```python
from build123d import *

# Parameters (mm, degrees)
F0_W     = 10
F0_H     = 20
F1_ANGLE = 180
F2_R     = 0.6542669189
F2_R_2   = 0.5762174249
F2_R_3   = 1.2390393019
F2_R_4   = 1.4098966941
F2_R_5   = 0.189897881
F2_R_6   = 0.6151811848
F2_R_7   = 0.7778029264
F2_R_8   = 0.6623255224
F2_R_9   = 0.6070903234
F2_R_10  = 0.7783808961
F2_R_11  = 0.265053414
F2_R_12  = 0.5177294077
F2_R_13  = 0.5684145952
F2_R_14  = 0.5786464401
F4_DEPTH = 1


# Not quite as in the source:
# - the program builds the solid bodies; features that only make, move or delete a surface that nothing else refers to are left out


with BuildPart() as f1:
    # F0 (on Front) → F1 (revolve)
    with BuildSketch(Plane.XZ):
        with Locations((5, 10)):
            Rectangle(F0_W, F0_H)
        with BuildLine():
            Line((10, 0), (0, 0))
            ThreePointArc((0, 0), (2.9289321881, -7.0710678119), (10, -10))
            Line((10, -10), (10, 0))
        make_face()
        with BuildLine():
            ThreePointArc((10, 30), (2.9289321881, 27.0710678119), (0, 20))
            Line((0, 20), (10, 20))
            Line((10, 20), (10, 30))
        make_face()
    revolve(axis=Axis((10, 0, 10), (0, 0, -1)), revolution_arc=F1_ANGLE)

    # F2 (on face) → F4 (join)
    with BuildSketch(Plane.XZ):
        with Locations((5.6774760596, 22.7308552712)):
            Circle(F2_R)
        with Locations((16.3127072155, 20.606238395)):
            Circle(F2_R_2)
        with Locations((3.6300569773, 15.6070627272)):
            Circle(F2_R_3)
        with Locations((16.507089138, 4.3547041714)):
            Circle(F2_R_4)
        with Locations((3.5698860884, 7.9049132764)):
            Circle(F2_R_5)
        with Locations((16.3283385336, 16.4442379028)):
            Circle(F2_R_6)
        with Locations((3.9457399398, -4.0635056794)):
            Circle(F2_R_7)
        with Locations((3.19618918, 2.172768116)):
            Circle(F2_R_8)
        with Locations((11.4412605762, 28.0772857368)):
            Circle(F2_R_9)
        with Locations((6.0145035386, 27.1478407085)):
            Circle(F2_R_10)
        with Locations((15.0091275573, 23.699901998)):
            Circle(F2_R_11)
        with Locations((12.4958753586, -4.2460225523)):
            Circle(F2_R_12)
        with Locations((13.1159704179, -1.4507770538)):
            Circle(F2_R_13)
        with Locations((17.5564400852, 11.2137598917)):
            Circle(F2_R_14)
    extrude(amount=F4_DEPTH)


solid = f1.part
```
Input: part model. Units: mm. Frame: model coordinates. A direction names the side the tool comes from. Give positions to 0.01 mm unless a question says otherwise; leave off trailing zeros. Loops run counter-clockwise (first coordinate to the right, second up) from the corner with the lowest first, then second, coordinate; pieces in that order, holes last.
1) Reachability of faces 1 (the cylindrical face through (5.91, -0.49, 27.92)), 2 (the flat face through (3, -1, 2)) from +Z, -Z, +X, -X, +Y, -Y: full face, straight path, thin tool, end or side. Return the list, or none.
A:
face 1: -Y
face 2: +Z, -Z, +X, -X, -Y
2) Section query B-B on z = 13. Return the cut outline in (x, y), and give its area (3 significant figures).
A:
outline: (0, 0) - (20, 0) arc R10 ccw to start
area: 157 mm2
3) Section query C-C on y = 3.5. Return the cut outline in (x, z) (1 decimal).
A:
outline: (0.6, 0) arc R9.4 ccw to (19.4, 0) - (19.4, 20) arc R9.4 ccw to (0.6, 20) - close
4) Section query A-A on x = 10. Return the cut outline in (y, z).
A:
outline: (0, -10) arc R10 ccw to (10, 0) - (10, 20) arc R10 ccw to (0, 30) - close
5) Contact query for flat-ended pins moving along their axis: pin 1 (1.5 mm diameter, centred on x = 10, z = 20, fed in from -Y); pin 2 (10 mm diameter, centred on x = 15.5, z = 2, fed in from +Y); pin 3 (5 mm diameter, centred on x = 16, z = 5, fed in from +Y). Output: stop coordinate, or through.
A:
pin 1: stops at y = 0
pin 2: stops at y = 9.99
pin 3: stops at y = 9.37
6) Mould query, pull axis X, two halves, no side actions, for faces 3 (the flat face through (4, -1, 16)), 4 (the cylindrical face through (12.974, -0.493, -4.444)), 5 (the cylindrical face through (12.548, -0.493, -1.426)), 6 (the cylindrical face through (16.612, -0.493, 15.898)). Classes: released by +X, released by -X, zero draft, split by the parting line, or undercut.
A:
face 3: zero draft
face 4: undercut
face 5: split by the parting line
face 6: undercut
7) Section query D-D on z = -0.5. Return the cut outline in (x, y), and give its area (3 significant figures).
A:
outline: (0.01, 0) - (19.99, 0) arc R9.99 ccw to start
area: 157 mm2
8) Line query: L1, parallel to Z at x = 8, y = 8.5; L2, parallel to Z at x = 16.75, y = 4.25; L3, parallel to X at y = 3.5, z = 22.5. Output: solid intervals per line, ascending.
A:
L1: z = -4.87 to 24.87
L2: z = -6.03 to 26.03
L3: x = 0.97 to 19.03
